Geometry: final body of the model. Coordinates: model frame, mm. Face numbers are marked on the shaded views. Give positions to 0.01 mm unless a question says otherwise; leave off trailing zeros. Write each loop counter-clockwise with the first axis right and the second up, starting at its lowest first coordinate (ties: lowest second). Pieces come first, ordered by that corner, then holes. Notation, with made-up numbers: M 55,35.25 L 98,35.25 A31 cw 98,70.25 Z; hole C 87.5,-37.5 d9. An arc over 180 degrees is marked long. Use a Markdown table: item, result. Add a question column.
(1) Cut plane D-D (y = 45.5). State how many separate pieces and enclosed holes the cut face has, plus the area to 3 significant figures.
(2) Cut plane B-B (x = -20.5). Output: boundary loops of the cut face in (y, z).
(3) Draft query along Z for the marked faces 1, 2 and 3. Return one class per face: released by +Z, released by -Z, zero draft, split by the parting line, or undercut.
(4) Pin query (flat end, axial travel): pin 1 Ø3 at (x, z) = (-20.27, 18.84) entering from -Y; pin 2 Ø1 at (x, y) = (-4, 46) entering from -Z. Return the tip coordinate at first contact, or that it passes through.
(5) Cut plane C-C (z = 19). Output: boundary loops of the cut face in (x, y).
(6) Cut plane A-A (z = 17). Output: boundary loops of the cut face in (x, y).
(7) Material intervals for L1, parallel to X at y = 44.65, z = 19; L2, parallel to X at y = 45.7, z = 20.5; L3, parallel to Z at x = -3.5, y = 45.15, sorted ascending.
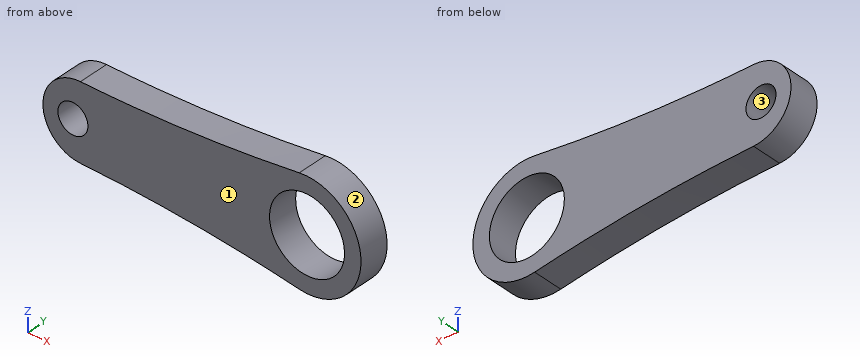
```python
from build123d import *

# Parameters (mm, degrees)
CROQUIS1_R              = 2.5
CROQUIS1_R_2            = 1
SALIENTE_EXTRUIR1_DEPTH = 2
REDONDEO1_R             = 101


with BuildPart() as part:
    # Croquis1 → Saliente-Extruir1 (new body)
    with BuildSketch(Plane(origin=(0, 44.435642752, 0), x_dir=(1, 0, 0), z_dir=(0, 1, 0))):
        with BuildLine():
            Line((-19.765786092, -16.344915397), (-7.245908087, -16.344915397))
            ThreePointArc((-7.245908087, -16.344915397), (-1.055541318, -18.844915397), (-7.245908087, -21.344915397))
            Line((-7.245908087, -21.344915397), (-19.765786092, -21.344915397))
            ThreePointArc((-19.765786092, -21.344915397), (-22.265786092, -18.844915397), (-19.765786092, -16.344915397))
        make_face()
        with Locations(Location((-4.655541318, -18.844915397, 0), (0, 0, 270))):
            Circle(CROQUIS1_R, mode=Mode.SUBTRACT)
        with Locations(Location((-20.265786092, -18.844915397, 0), (0, 0, 270))):
            Circle(CROQUIS1_R_2, mode=Mode.SUBTRACT)
    extrude(amount=SALIENTE_EXTRUIR1_DEPTH)

    # Redondeo1
    redondeo1_edges = [part.edges().sort_by_distance(p)[0] for p in [
        (-7.245908087, 45.435642752, 16.344915397),
        (-7.245908087, 45.435642752, 21.344915397),
    ]]
    fillet(redondeo1_edges, radius=REDONDEO1_R)


solid = part.part
```
Answer list:
| question | item | result |
|---|---|---|
| 1 | separate pieces | 1 |
| 1 | enclosed holes | 2 |
| 1 | area | 94.4 mm² |
| 2 | outline | M 44.44,16.46 L 46.44,16.46 L 46.44,17.87 L 44.44,17.87 Z; M 44.44,19.82 L 46.44,19.82 L 46.44,21.23 L 44.44,21.23 Z |
| 3 | face 1 | zero draft |
| 3 | face 2 | split by the parting line |
| 3 | face 3 | undercut |
| 4 | pin 1 | y = 44.44 |
| 4 | pin 2 | z = 15.25 |
| 5 | outline | M -22.26,44.44 L -21.25,44.44 L -21.25,46.44 L -22.26,46.44 Z; M -19.28,44.44 L -7.15,44.44 L -7.15,46.44 L -19.28,46.44 Z; M -2.16,44.44 L -1.06,44.44 L -1.06,46.44 L -2.16,46.44 Z |
| 6 | outline | M -21.45,44.44 L -6.34,44.44 L -6.34,46.44 L -21.45,46.44 Z; M -2.97,44.44 L -1.56,44.44 L -1.56,46.44 L -2.97,46.44 Z |
| 7 | L1 | -22.26 to -21.25, -19.28 to -7.15, -2.16 to -1.06 |
| 7 | L2 | -21.64 to -6.53, -2.78 to -1.46 |
| 7 | L3 | 15.44 to 16.63, 21.06 to 22.25 |
